Geometry check sheet. Reference: the model listing, model coordinates, mm. A direction names the side the tool comes from. Give positions to 0.01 mm unless a question says otherwise; leave off trailing zeros. Order: outer loops, then holes, each group sorted by start corner. A loop starts at its lowest first (then second) coordinate and runs counter-clockwise, first axis right, second up. Notation, with made-up numbers: M 31.25,77 L 79.25,77 A25 ccw 79.25,98 Z; hole C 53.5,-7.75 d5. An arc over 180 degrees is marked long. Answer as CSV lines item,"result". Start each with the question number.
```python
from build123d import *

# Parameters (mm, degrees)
SKETCH1_W           = 6.477
SKETCH1_H           = 2.54
BOSS_EXTRUDE1_DEPTH = 0.5
SKETCH2_W           = 6.477
SKETCH2_H           = 0.762
SKETCH2_W_2         = 18.161
BOSS_EXTRUDE2_DEPTH = 10.16


with BuildPart() as part:
    # Sketch1 → Boss-Extrude1 (new body)
    with BuildSketch(Plane(origin=(0, 0, 0), x_dir=(1, 0, 0), z_dir=(0, 1, 0))):
        Polygon((-18.161, -12.7), (18.161, -12.7), (18.161, 0), (0, 0), (0, 12.7), (-18.161, 12.7), align=None)
        with Locations((-9.0805, 1.27)):
            Rectangle(SKETCH1_W, SKETCH1_H, mode=Mode.SUBTRACT)
    extrude(amount=BOSS_EXTRUDE1_DEPTH)

    # Sketch2 → Boss-Extrude2 (add)
    with BuildSketch(Plane(origin=(0, 0.5, 0), x_dir=(1, 0, 0), z_dir=(0, 1, 0))):
        with Locations((-9.0805, -0.381)):
            Rectangle(SKETCH2_W, SKETCH2_H)
        with Locations((9.0805, -0.381)):
            Rectangle(SKETCH2_W_2, SKETCH2_H)
    extrude(amount=BOSS_EXTRUDE2_DEPTH)


solid = part.part
```
Item 1: Depth check by flat-ended pin: pin 1 Ø0.6 at (y, z) = (0, -9) entering from +X; pin 2 Ø3 at (x, z) = (-9.5, 3.5) entering from +Y; pin 3 Ø3 at (x, y) = (7.5, 4.5) entering from +Z. Enter the tip coordinate at first touch or a pass-through.
Item 2: Access from +Z, -Z, +X, -X, +Y, -Y to the whole of each face (thin tool, end or side, straight path). Record for faces 1 (the face through (-9, 6, 0.762)), 2 (the face through (-4, 0, 3)).
Item 3: Section check D-D on z = 5. Record the boundary of the cut face in (x, y).
Item 4: Scan lines: line 1 along Z through (x, y) = (9, 6.5); line 2 along Y through (x, z) = (-2, 2.75). Record each from-to range of solid material in increasing order.
Item 5: Section check A-A on y = 5.5. Record the boundary of the cut face in (x, z), then the cut area to 3 significant figures.
Item 6: Section check C-C on x = 15. Record the boundary of the cut face in (y, z), then the cut area to 3 significant figures.
Item 7: Section check B-B on z = -1.5. Record the boundary of the cut face in (x, y).
Numbers:
1,pin 1,"x = 0"
1,pin 2,"y = 0.5"
1,pin 3,"z = 0.76"
2,face 1,"+Z, +X, -X, +Y"
2,face 2,"+Z, -Z, +X, -X, -Y"
3,outline,"M -18.16,0 L 18.16,0 L 18.16,0.5 L -18.16,0.5 Z"
4,line 1,"0 to 0.76"
4,line 2,"0 to 0.5"
5,outline,"M -12.32,0 L -5.84,0 L -5.84,0.76 L -12.32,0.76 Z; M 0,0 L 18.16,0 L 18.16,0.76 L 0,0.76 Z"
5,area,"18.8 mm2"
6,outline,"M 0,0 L 10.66,0 L 10.66,0.76 L 0.5,0.76 L 0.5,12.7 L 0,12.7 Z"
6,area,"14.1 mm2"
7,outline,"M -18.16,0 L -12.32,0 L -12.32,0.5 L -18.16,0.5 Z; M -5.84,0 L 0,0 L 0,0.5 L -5.84,0.5 Z"
